Autodesk Inventor part; units mm, degrees
ref_plane "YZ Plane" through (0, 0, 0) normal (1, 0, 0) x (0, 1, 0)
ref_plane "XZ Plane" through (0, 0, 0) normal (0, 1, 0) x (-1, 0, 0)
ref_plane "XY Plane" through (0, 0, 0) normal (0, 0, 1) x (1, 0, 0)
sketch "Esboço1" plane through (0, 0, 0) normal (0, 0, 1) x (1, 0, 0)
  line L0 (-20, -35.65) -> (20, -35.65)
  line L1 (20, -35.65) -> (20, 35.65)
  line L2 (20, 35.65) -> (-20, 35.65)
  line L3 (-20, 35.65) -> (-20, -35.65)
  line L4 (-20, 35.65) -> (20, 35.65)
  circle A0 centre (0, 25.65) radius 5 construction
  circle A1 centre (0, 25.65) radius 28 construction
  circle A2 centre (0, 25.65) radius 74 construction
  line L5 (-20, 6.0541) -> (20, 6.0541) construction
  line L6 (-20, -48.35) -> (20, -48.35) construction
  line L7 (-103.6, 0) -> (103.6, 0) construction
  line L8 (0, -77.95) -> (0, 129.25) construction
  line L9 (-20, 24.932) -> (20, 35.65)
  point P0 (0, 0)
  dimension "d0" = 71.3
  dimension "d1" = 40
  dimension "d41" = 10
  dimension "d42" = 61.3
  dimension "d43" = 56
  dimension "d45" = 84
  dimension "d49" = 15
  dimension "d58" = 10
extrude "Extrusão1" add sketch "Esboço1" along normal mid plane 10
extrude "Extrusão4" cut sketch "Esboço1" along normal through all both and the other way through all contours L3 L2 L9
sketch "Esboço2" plane through (-20, -35.65, -5) normal (0, -1, 0) x (1, 0, 0)
  line L0 (40, 10) -> (40, 0)
  line L1 (40, 5) -> (0, 5) construction
  line L2 (0, 0) -> (0, 10)
  line L3 (0, 0) -> (0, 10)
  line L4 (40, 0) -> (40, 10)
  line L5 (0, 10) -> (40, 10) construction
  line L6 (20, 10) -> (20, 0) construction
  line L7 (40, 0) -> (0, 0) construction
  point P0 (20, 5)
  point P1 (7.5, 5)
  point P2 (32.5, 5)
  dimension "d9" = 7.5
  dimension "d10" = 7.5
  dimension "d37" = 25
hole "Furo1" at (-12.5, -35.65, 0) at (12.5, -35.65, 0) direction (0, 1, 0) diameter 3.242 depth 15 tip angle 118
sketch "Esboço3" plane through (0, 0, 5) normal (0, 0, 1) x (1, 0, 0)
  point P0 (0, 0)
  point P1 (0, 37.5)
  point P2 (0, 25.65)
hole "Furo2" [suppressed]
sketch "Esboço6" plane through (20, 35.65, 5) normal (-0.258819, 0.9659258, 0) x (0.9659258, 0.258819, 0)
  line L0 (0, 0) -> (0, 10) construction
  line L1 (0, 5) -> (-41.411, 5) construction
  line L2 (-41.411, 0) -> (-41.411, 10) construction
  line L3 (-20.7055, 5) -> (-20.7055, 0) construction
  point P0 (-28.5454, 5)
  point P1 (-30.7055, 5)
  point P2 (-10.7055, 5)
  dimension "d50" = 20
hole "Furo3" at (-9.6593, 27.7028, 0) direction (0.258819, -0.9659258, 0) diameter 3.242 depth 15 tip angle 118 countersink diameter 10 countersink angle 90
properties part number "GRJ-03-115" material "Fenolite OR"
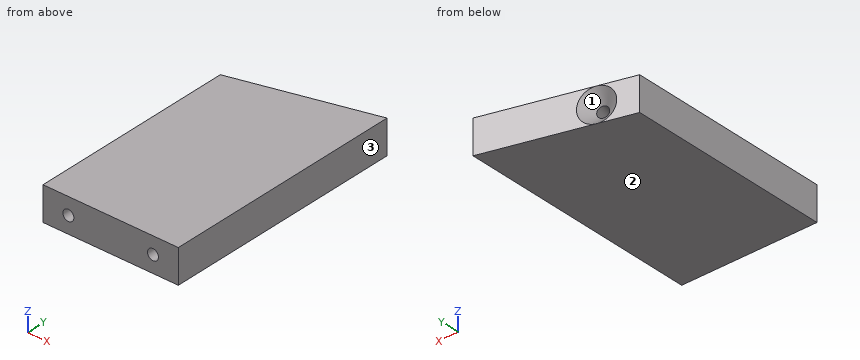
Design review of the part built by this model. Coordinates are the model's own, in mm. Face numbers are marked on the shaded views. Round coordinates to 2 decimals unless told otherwise and drop trailing zeros. Write each loop counter-clockwise with the first axis right and the second up, starting at its lowest first coordinate (ties: lowest second). Pieces come first, ordered by that corner, then holes.
Item 1: We need section A-A on y = -30. Write out the cut boundary in (x, z).
Item 2: The part is to be moulded in two halves that separate along Z. For the marked faces 1, 2 and 3, say which applies: +Z half, -Z half, draft (parallel to the pull), parting line (faces both ways), or undercut.
Item 3: Clearance check with flat-ended pins moving along their axes: pin 1 Ø3.5 at (x, z) = (12.5, 0) entering from +Y; pin 2 Ø1.5 at (x, z) = (-16, 1) entering from +Y; pin 3 Ø3 at (x, z) = (1, -1.5) entering from +Y; pin 4 Ø5 at (x, z) = (-12.5, 0) entering from -Y. State where each tip first meets the part, or that it passes through.
Item 4: For probe 1 along X at (y, z) = (-31.25, 0); probe 2 along Z at (x, y) = (12.5, -30.5); probe 3 along Z at (x, y) = (12, -24), list the stretches that pass through material, from the lowest coordinate up.
Item 5: We need section B-B on x = -3. Write out the cut boundary in (y, z), and give its area (3 significant figures).
Returned:
1. outline: (-20, -5) - (20, -5) - (20, 5) - (-20, 5) - close; hole circle Ø3.24 at (-12.5, 0); hole circle Ø3.24 at (12.5, 0)
2. face 1: undercut
2. face 2: -Z half
2. face 3: draft
3. pin 1: stops at y = 34.11
3. pin 2: stops at y = 26.2
3. pin 3: stops at y = 30.96
3. pin 4: stops at y = -35.65
4. probe 1: x = -20 to -14.12, -10.88 to 10.88, 14.12 to 20
4. probe 2: z = -5 to -1.62, 1.62 to 5
4. probe 3: z = -5 to -1.54, 1.54 to 5
5. outline: (-35.65, -5) - (29.49, -5) - (29.49, 5) - (-35.65, 5) - close
5. area: 651 mm2
